Could you check a few things on this model? Use its own coordinates, in mm. Give positions to 0.01 mm unless a question says otherwise; leave off trailing zeros. Loops run counter-clockwise (first coordinate to the right, second up) from the corner with the lowest first, then second, coordinate; pieces in that order, holes last.
1. Thinking about a two-plate mould opening in X: for faces 1 (the flat face through (-7.605, 3.352, -3.724)), 2 (the flat face through (3.5, -3, 0)), 3 (the cylindrical face through (-11.829, 2.183, -5.822)), 4 (the cylindrical face through (-14.7, -7.17, 2.99)), which applies, +X half, -X half, draft (parallel to the pull), parting line (faces both ways), or undercut?
2. I need wall thicknesses on line 1 along X through (y, z) = (-2, 3); line 2 along Z through (x, y) = (-5, 0.25); line 3 along X through (y, z) = (0.25, 1.75). Which ranges of each line are inside material? Lowest first, please.
3. For P1, Ø4, axis at x = -6.5, y = 2, coming from the -Z side; P2, Ø8, axis at x = 15.5, z = 3, coming from the -Y side; P3, Ø6, axis at x = -10, z = 3.5, coming from the -Y side, each with a flat end and sliding along its axis, tell me the tip position at first contact or that it passes through.
4. Imagine slicing it at A-A (x = -5). List the corners of the cut face in (y, z) for me, plus the area to 3 significant figures.
```python
from build123d import *

# Parameters (mm, degrees)
BASEHEAD_DEPTH      = 3.5
THDSCHPAT_COUNT     = 30
THDSCHPAT_PITCH     = 0.8
BOSS_EXTRUDE1_DEPTH = 5
FILLET1_R           = 1
SKETCH2_R           = 2.210363486
CUT_EXTRUDE1_DEPTH  = 23


with BuildPart() as part:
    # BaseHeadSke → BaseHead (new body)
    with BuildSketch(Plane(origin=(0, 0, 0), x_dir=(0, 0, -1), z_dir=(1, 0, 0))):
        Polygon((0, 4.618802154), (-4, 2.309401077), (-4, -2.309401077), (0, -4.618802154), (4, -2.309401077), (4, 2.309401077), align=None)
    extrude(amount=BASEHEAD_DEPTH)

    # HeadChamferSke → HeadChamfer (revolve, cut)
    with BuildSketch(Plane.XY):
        Polygon((0, 4.618802154), (0, 4), (0.35726559, 4.618802154), align=None)
    revolve(axis=Axis((0, 0, 0), (1, 0, 0)), mode=Mode.SUBTRACT)

    # BodySke → BaseBody (revolve)
    with BuildSketch(Plane.XY, mode=Mode.PRIVATE) as basebody_sk:
        Polygon((0, 0), (0, 2.5), (28.055, 2.5), (28.5, 2.055), (28.5, 0), align=None)
    revolve(basebody_sk.sketch.rotate(Axis((0, 0, 0), (1, 0, 0)), 90), axis=Axis((0, 0, 0), (1, 0, 0)))

    # ThdSchSke → ThreadSchematic (revolve, cut)
    with BuildSketch(Plane.XY, mode=Mode.PRIVATE) as threadschematic_sk:
        Polygon((27.255, 3.01384174), (27.255, 2.5), (27.51192087, 2.055), (27.76884174, 2.5), (27.76884174, 3.01384174), align=None)
    threadschematic = revolve(threadschematic_sk.sketch.rotate(Axis((0, 0, 0), (1, 0, 0)), 90), axis=Axis((0, 0, 0), (1, 0, 0)), mode=Mode.SUBTRACT)

    # ThdSchPat: ThreadSchematic ×30
    with Locations(*[(-i * THDSCHPAT_PITCH, 0, 0) for i in range(1, THDSCHPAT_COUNT)]):
        add(threadschematic, mode=Mode.SUBTRACT)

    # Sketch1 → Boss-Extrude1 (add, symmetric)
    with BuildSketch(Plane(origin=(0, 0, 0), x_dir=(-1, 0, 0), z_dir=(0, -0.8660254037844388, -0.49999999999999983))):
        with BuildLine():
            Line((0, 7.400996674), (15, 7.400996674))
            Line((15, 7.400996674), (15, 4.900996674))
            Line((15, 4.900996674), (0, 4.900996674))
            Line((0, 4.900996674), (0, 0))
            Line((0, 0), (0, -4.909542525))
            Line((0, -4.909542525), (15, -4.909542525))
            Line((15, -4.909542525), (15, -7.409542525))
            Line((15, -7.409542525), (-0.5, -7.409542525))
            ThreePointArc((-0.5, -7.409542525), (-2.621320344, -6.530862869), (-3.5, -4.409542525))
            Line((-3.5, -4.409542525), (-3.5, 4.400996674))
            ThreePointArc((-3.5, 4.400996674), (-2.621320344, 6.522317018), (-0.5, 7.400996674))
            Line((-0.5, 7.400996674), (0, 7.400996674))
        make_face()
    extrude(amount=BOSS_EXTRUDE1_DEPTH, both=True)

    # Fillet1
    fillet1_edges = [part.edges().sort_by_distance(p)[0] for p in [
        (-15, 1.250355756, 7.834320303),
        (-15, 7.405625356, -2.826919378),
        (-15, -7.409898282, 2.834320303),
        (-15, -1.254628682, -7.826919378),
    ]]
    fillet(fillet1_edges, radius=FILLET1_R)

    # Sketch2 → Cut-Extrude1 (cut)
    with BuildSketch(Plane(origin=(0, -3.704771263, 6.416852057), x_dir=(1, 0, 0), z_dir=(0, -0.49999999999999983, 0.8660254037844387))):
        with Locations(Location((-9.867615043, 0, 0), (0, 0, 270))):
            Circle(SKETCH2_R)
    extrude(amount=-CUT_EXTRUDE1_DEPTH, mode=Mode.SUBTRACT)


solid = part.part
```
Derived:
1. face 1: draft
1. face 2: +X half
1. face 3: undercut
1. face 4: -X half
2. line 1: x = 0 to 3.5
2. line 2: z = -8.4 to -5.51, 5.81 to 8.7
2. line 3: x = 0 to 28.5
3. P1: stops at z = -8.55
3. P2: stops at y = -2.5
3. P3: stops at y = -8.03
4. outline: (-8.03, 3.92) - (-6.78, 1.75) - (1.88, 6.75) - (0.63, 8.92) - close; (-1.88, -6.74) - (-0.63, -8.91) - (8.03, -3.91) - (6.78, -1.74) - close
4. area: 50.0 mm2
